from build123d import *

# Parameters (mm, degrees)
CYLINDER001_R     = 1.75
CYLINDER001_DEPTH = 10
CYLINDER_R        = 1.75
CYLINDER_DEPTH    = 10
BOX_W             = 40
BOX_H             = 15
BOX_DEPTH         = 3
FILLET001_R       = 0.5


with BuildPart() as cilindro001:
    # Cylinder001 → Cylinder001 (new body)
    with BuildSketch(Plane(origin=(29.5, 7.5, -4), x_dir=(1, 0, 0), z_dir=(0, 0, 1))):
        Circle(CYLINDER001_R)
    extrude(amount=CYLINDER001_DEPTH)


with BuildPart() as cilindro:
    # Cylinder → Cylinder (new body)
    with BuildSketch(Plane(origin=(11.5, 7.5, -4), x_dir=(1, 0, 0), z_dir=(0, 0, 1))):
        Circle(CYLINDER_R)
    extrude(amount=CYLINDER_DEPTH)


with BuildPart() as fillet001:
    # Box → Box (new body)
    with BuildSketch(Plane.XY):
        with Locations((20, 7.5)):
            Rectangle(BOX_W, BOX_H)
    extrude(amount=BOX_DEPTH)

    # Cut: cut Cilindro
    add(cilindro.part, mode=Mode.SUBTRACT)

    # Cut001: cut Cilindro001
    add(cilindro001.part, mode=Mode.SUBTRACT)

    # Fillet001
    fillet001_edges = [fillet001.edges().sort_by_distance(p)[0] for p in [
        (0, 0, 1.5),
        (0, 7.5, 3),
        (0, 15, 1.5),
        (40, 0, 1.5),
        (20, 0, 3),
        (20, 15, 3),
        (40, 7.5, 3),
        (40, 15, 1.5),
    ]]
    fillet(fillet001_edges, radius=FILLET001_R)


solid = fillet001.part
The listing builds one solid part. Answer for the finished solid, in the listing's coordinates (mm). Give positions to 0.01 mm unless a question says otherwise; leave off trailing zeros. Write each loop counter-clockwise with the first axis right and the second up, starting at its lowest first coordinate (ties: lowest second). Pieces come first, ordered by that corner, then holes. Notation, with made-up numbers: (88, 39.5) -> (132, 39.5) arc R8 ccw to (132, 53.5) -> close; hole circle Ø1 at (44, 87.5). An arc over 180 degrees is marked (long way). One line per question, with ' | ' between items. Start each with the question number.
1. Find the intervals of material crossed by probe 1 along X at (y, z) = (7.5, 0.95); probe 2 along Y at (x, z) = (11.5, 0.8); probe 3 along X at (y, z) = (8.25, 2.1), in increasing order.
2. Section B-B (x = 29.5) is taken. Determine the outline of the cut face in (y, z), plus the area to 3 significant figures.
3. Section D-D (x = 12) is taken. Determine the outline of the cut face in (y, z), plus the area to 3 significant figures.
4. Section C-C (y = 6.5) is taken. Determine the outline of the cut face in (x, z).
5. For a pull along Y with two mould halves and no side action, classify faces 1 (the cylindrical face through (13.117, 6.83, 1.479)), 2 (the flat face through (40, 7, 1)), 3 (the flat face through (20, 15, 1)) as pulls with the +Y half, pulls with the -Y half, needs draft (parallel to the pull), parting line crosses it, or undercut.
6. Section A-A (z = 0.75) is taken. Determine the outline of the cut face in (x, y).
Response values:
1) probe 1: 0 to 9.75, 13.25 to 27.75, 31.25 to 40 | probe 2: 0 to 5.75, 9.25 to 15 | probe 3: 0 to 9.92, 13.08 to 27.92, 31.08 to 40
2) outline: (0, 0) -> (5.75, 0) -> (5.75, 3) -> (0.5, 3) arc R0.5 ccw to (0, 2.5) -> close; (9.25, 0) -> (15, 0) -> (15, 2.5) arc R0.5 ccw to (14.5, 3) -> (9.25, 3) -> close | area: 34.4 mm2
3) outline: (0, 0) -> (5.82, 0) -> (5.82, 3) -> (0.5, 3) arc R0.5 ccw to (0, 2.5) -> close; (9.18, 0) -> (15, 0) -> (15, 2.5) arc R0.5 ccw to (14.5, 3) -> (9.18, 3) -> close | area: 34.8 mm2
4) outline: (0, 0) -> (10.06, 0) -> (10.06, 3) -> (0.5, 3) arc R0.5 ccw to (0, 2.5) -> close; (12.94, 0) -> (28.06, 0) -> (28.06, 3) -> (12.94, 3) -> close; (30.94, 0) -> (40, 0) -> (40, 2.5) arc R0.5 ccw to (39.5, 3) -> (30.94, 3) -> close
5) face 1: undercut | face 2: needs draft | face 3: pulls with the +Y half
6) outline: (0, 0.5) arc R0.5 ccw to (0.5, 0) -> (39.5, 0) arc R0.5 ccw to (40, 0.5) -> (40, 14.5) arc R0.5 ccw to (39.5, 15) -> (0.5, 15) arc R0.5 ccw to (0, 14.5) -> close; hole circle Ø3.5 at (11.5, 7.5); hole circle Ø3.5 at (29.5, 7.5)
